```python
from build123d import *

# Parameters (mm, degrees)
SKETCH1_W           = 40
SKETCH1_H           = 25
BOSS_EXTRUDE1_DEPTH = 20
CUT_EXTRUDE1_DEPTH  = 33.398148095
HOLE1_D             = 4.4
HOLE2_D             = 4.4


with BuildPart() as part:
    # Sketch1 → Boss-Extrude1 (new body)
    with BuildSketch(Plane.XY.offset(20)):
        with Locations((0, -3.3)):
            Rectangle(SKETCH1_W, SKETCH1_H)
    extrude(amount=-BOSS_EXTRUDE1_DEPTH)

    # Sketch2 → Cut-Extrude1 (cut, through all)
    with BuildSketch(Plane(origin=(0, 0, 0), x_dir=(-1, 0, 0), z_dir=(0, 0, -1))):
        with BuildLine():
            Line((10, 9.2), (-10, 9.2))
            Line((-10, 9.2), (-10, 0))
            ThreePointArc((-10, 0), (0, -10), (10, 0))
            Line((10, 0), (10, 9.2))
        make_face()
    extrude(amount=-CUT_EXTRUDE1_DEPTH, mode=Mode.SUBTRACT)

    # Hole1 (through all)
    with Locations(Plane(origin=(0, 9.2, 0), x_dir=(-1, 0, 0), z_dir=(0, 1, 0))):
        with Locations((15, 10)):
            Hole(HOLE1_D / 2)

    # Hole2 (through all)
    with Locations(Plane(origin=(0, 9.2, 0), x_dir=(-1, 0, 0), z_dir=(0, 1, 0))):
        with Locations((-15, 10)):
            Hole(HOLE2_D / 2)


solid = part.part
```
The listing builds one solid part. Answer for the finished solid, in the listing's coordinates (mm). A direction names the side the tool comes from. Coordinates: 2 decimals unless noted, no trailing zeros. Write each loop counter-clockwise with the first axis right and the second up, starting at its lowest first coordinate (ties: lowest second). Pieces come first, ordered by that corner, then holes. Notation, with made-up numbers: (5, 43) - (33, 43) arc R26 ccw to (33, 68) - close; hole circle Ø7 at (32.5, 87). An arc over 180 degrees is marked (long way). Return JSON: item names as keys, results as strings. Group by question number.
Q1. For a pull along X with two mould halves and no side action, classify faces 3 (the flat face through (0, -15.8, 10)), 4 (the flat face through (20, -3, 10)), 5 (the cylindrical face through (17.032, -3.475, 9.157)) as +X half, -X half, draft (parallel to the pull), parting line (faces both ways), or undercut.
Q2. Which of the six approach directions +Z, -Z, +X, -X, +Y, -Y give full straight-line access (tool end or side, diameter ignored) to faces 1 (the flat face through (14.9, 9.2, 12.4)), 2 (the flat face through (10, 5, 10))?
Q3. Flat-ended cylindrical pins translate along their axes: pin 1 Ø12 at (x, z) = (-3, 18) entering from +Y; pin 2 Ø4 at (x, z) = (-15, 10) entering from +Y. Find the tip coordinate at first contact, or state that the pin passes through.
Q4. The part is cut by section A-A on x = 15. Write down the section's boundary in (y, z).
Q5. The part is cut by section D-D on z = 2.25. Write down the section's boundary in (x, y), and give its area (3 significant figures).
Q6. Find the intervals of material crossed by line 1 along X through (y, z) = (3.5, 6.75); line 2 along Z through (x, y) = (-15, 2.75); line 3 along X through (y, z) = (-2, 8.75), in increasing order. Write a range as [from, to].
Q7. The part is cut by section C-C on y = -13. Write down the section's boundary in (x, z), and give its area (3 significant figures).
Q8. The part is cut by section B-B on y = 0.75. Write down the section's boundary in (x, z), and give its area (3 significant figures).
Evaluation:
{
 "1": {"face 3": "draft", "face 4": "+X half", "face 5": "undercut"},
 "2": {"face 1": "+Z, -Z, +X, -X, +Y", "face 2": "+Z, -Z, +Y"},
 "3": {"pin 1": "stops at y = -4.36", "pin 2": "passes through"},
 "4": {"outline": "(-15.8, 0) - (9.2, 0) - (9.2, 7.8) - (-15.8, 7.8) - close; (-15.8, 12.2) - (9.2, 12.2) - (9.2, 20) - (-15.8, 20) - close"},
 "5": {"outline": "(-20, -15.8) - (20, -15.8) - (20, 9.2) - (10, 9.2) - (10, 0) arc R10 cw to (-10, 0) - (-10, 9.2) - (-20, 9.2) - close", "area": "659 mm2"},
 "6": {"line 1": "x = [-20, -10], [10, 20]", "line 2": "z = [0, 7.8], [12.2, 20]", "line 3": "x = [-20, -16.81], [-13.19, -9.8], [9.8, 13.19], [16.81, 20]"},
 "7": {"outline": "(-20, 0) - (20, 0) - (20, 20) - (-20, 20) - close; hole circle Ø4.4 at (-15, 10); hole circle Ø4.4 at (15, 10)", "area": "770 mm2"},
 "8": {"outline": "(-20, 0) - (-10, 0) - (-10, 20) - (-20, 20) - close; (10, 0) - (20, 0) - (20, 20) - (10, 20) - close; hole circle Ø4.4 at (-15, 10); hole circle Ø4.4 at (15, 10)", "area": "370 mm2"}
}
